```python
from build123d import *

# Parameters (mm, degrees)
BOSS_EXTRUDE1_DEPTH = 16
SKETCH4_R           = 11
BOSS_EXTRUDE5_DEPTH = 45
SKETCH8_R           = 12.5
BOSS_EXTRUDE8_DEPTH = 50
SKETCH11_R          = 12.5
CUT_EXTRUDE1_DEPTH  = 50
SKETCH12_R          = 17.5
CUT_EXTRUDE2_DEPTH  = 5
BOSS_EXTRUDE9_DEPTH = 6
RIB4_REACH          = 156.758
SKETCH16_WALL_W     = 366.24251427
SKETCH16_WALL_H     = 10


with BuildPart() as part:
    # Sketch2 → Boss-Extrude1 (new body)
    with BuildSketch(Plane(origin=(0, 0, 0), x_dir=(1, 0, 0), z_dir=(0, 1, 0))):
        with BuildLine():
            Line((0, 19), (0, 30))
            ThreePointArc((0, 30), (-30, 0), (0, -30))
            Line((0, -30), (0, -19))
            ThreePointArc((0, -19), (-19, 0), (0, 19))
        make_face()
    extrude(amount=BOSS_EXTRUDE1_DEPTH)



with BuildPart() as body_2:
    # Sketch4 → Boss-Extrude5 (new body)
    with BuildSketch(Plane(origin=(0, 0, 0), x_dir=(1, 0, 0), z_dir=(0, 1, 0))):
        with BuildLine():
            Line((-122.5, 25), (-105.941325388, 25))
            ThreePointArc((-105.941325388, 25), (-80.941325388, 0), (-105.941325388, -25))
            Line((-105.941325388, -25), (-122.5, -25))
            Line((-122.5, -25), (-122.5, 25))
        make_face()
        with Locations(Location((-105.941325388, 0, 0), (0, 0, 90))):
            Circle(SKETCH4_R, mode=Mode.SUBTRACT)
    extrude(amount=BOSS_EXTRUDE5_DEPTH)

    # Sketch8 → Boss-Extrude8 (add)
    with BuildSketch(Plane.XY.offset(25)):
        with Locations((-122.5, 22.5)):
            Circle(SKETCH8_R)
        with BuildLine():
            ThreePointArc((-122.5, 45), (-145, 22.5), (-122.5, 0))
            Line((-122.5, 0), (-122.5, 45))
        make_face()
        with BuildLine():
            ThreePointArc((-122.5, 35), (-135, 22.5), (-122.5, 10))
            Line((-122.5, 10), (-122.5, 35))
        make_face()
        with BuildLine():
            Line((-122.5, 35), (-122.5, 10))
            ThreePointArc((-122.5, 10), (-113.661165235, 13.661165235), (-110, 22.5))
            ThreePointArc((-110, 22.5), (-113.661165235, 31.338834765), (-122.5, 35))
        make_face()
    extrude(amount=-BOSS_EXTRUDE8_DEPTH)

    # Sketch11 → Cut-Extrude1 (cut)
    with BuildSketch(Plane.XY.offset(25)):
        with Locations((-122.5, 22.5)):
            Circle(SKETCH11_R)
    extrude(amount=-CUT_EXTRUDE1_DEPTH, mode=Mode.SUBTRACT)

    # Sketch12 → Cut-Extrude2 (cut)
    with BuildSketch(Plane.XY.offset(25)):
        with Locations((-122.5, 22.5)):
            Circle(SKETCH12_R)
    extrude(amount=-CUT_EXTRUDE2_DEPTH, mode=Mode.SUBTRACT)


with BuildPart() as part_1:
    add(part.part)

    add(body_2.part)  # Boss-Extrude9 merges body 2
    # Sketch13 → Boss-Extrude9 (add)
    with BuildSketch(Plane(origin=(0, 0, 0), x_dir=(1, 0, 0), z_dir=(0, 1, 0))):
        with BuildLine():
            ThreePointArc((-105.941325388, 25), (-80.941325388, 0), (-105.941325388, -25))
            Line((-105.941325388, -25), (-2.825462558, -29.86664965))
            ThreePointArc((-2.825462558, -29.86664965), (-30, 0), (-2.825462558, 29.86664965))
            Line((-2.825462558, 29.86664965), (-105.941325388, 25))
        make_face()
    extrude(amount=BOSS_EXTRUDE9_DEPTH)

    # Sketch16 wall → Rib4 (add, up to next)
    with BuildSketch(Plane(origin=(-55.470662694, 23, 0), x_dir=(0.930830223145, -0.365451906112, 0), z_dir=(0.365451906112, 0.930830223145, 0)), mode=Mode.PRIVATE) as rib4_sk1:
        Rectangle(SKETCH16_WALL_W, SKETCH16_WALL_H)
    rib4_tool1 = extrude(rib4_sk1.sketch, amount=-RIB4_REACH, mode=Mode.PRIVATE) - part_1.part
    add(rib4_tool1.solids().sort_by_distance((-55.470662694, 23, 0))[0])


solid = part_1.part
```
Build history of the part. All positions in model axes, mm. A direction names the side the tool comes from. Give positions to 0.01 mm unless a question says otherwise; leave off trailing zeros. Loops run counter-clockwise (first coordinate to the right, second up) from the corner with the lowest first, then second, coordinate; pieces in that order, holes last. Notation, with made-up numbers: (67.5, 35.25) -> (104.5, 35.25) arc R18 cw to (104.5, 50.25) -> close; hole circle Ø6 at (26, 31). An arc over 180 degrees is marked (long way). One line per question, with ' | ' between items.
Q1. Cut at D-D, the plane z = 12.5. Write the cut outline in (x, y), plus the area to 3 significant figures.
Filled sheet:
outline: (-122.5, 0) -> (-14.31, 0) -> (-14.31, 16) -> (-27.27, 16) -> (-27.27, 6) -> (-84.29, 6) -> (-84.29, 45) -> (-122.5, 45) arc R22.5 ccw to start; hole circle Ø25 at (-122.5, 22.5) | area: 2,570 mm²
Q2. Tool access for faces 4 (the flat face through (-134, 28, -25)), 5 (the flat face through (-55, 6, -18)), 6 (the cylindrical face through (-105.81, 27.76, 22.54)), 7 (the cylindrical face through (-82.267, 25.227, 8.032)), 8 (the flat face through (-58, 14, 5)): list every direction of +Z, -Z, +X, -X, +Y, -Y with a clear straight run to the whole face (end or side of a thin tool).
Filled sheet:
face 4: -Z, -X, +Y, -Y | face 5: -Z, +Y | face 6: +Z | face 7: +Y | face 8: +Z, +Y
Q3. Drop flat-ended pins along their axis: pin 1 (4 mm diameter, centred on y = 35.5, z = -2.5, fed in from -X); pin 2 (1 mm diameter, centred on y = 24.5, z = -23, fed in from +X); pin 3 (13.5 mm diameter, centred on x = -50.5, y = 13.5, fed in from +Z); pin 4 (15 mm diameter, centred on x = -122.5, y = 22.5, fed in from +Z). Give the stop position or say it passes through.
Filled sheet:
pin 1: stops at x = -142.13 | pin 2: stops at x = -95.04 | pin 3: stops at z = 5 | pin 4: passes through
Q4. Cut at A-A, the plane x = -125. Write the cut outline in (y, z).
Filled sheet:
outline: (0.14, -25) -> (10.25, -25) -> (10.25, 20) -> (5.18, 20) -> (5.18, 25) -> (0.14, 25) -> close; (34.75, -25) -> (44.86, -25) -> (44.86, 25) -> (39.82, 25) -> (39.82, 20) -> (34.75, 20) -> close
Q5. Cut at B-B, the plane y = 8.5. Write the cut outline in (x, z).
Filled sheet:
outline: (-140.11, -25) -> (-105.94, -25) arc R25 ccw to (-81.45, -5) -> (-29.58, -5) arc R30 ccw to (0, -30) -> (0, -19) arc R19 cw to (0, 19) -> (0, 30) arc R30 ccw to (-29.58, 5) -> (-81.45, 5) arc R25 ccw to (-105.94, 25) -> (-112, 25) -> (-112, 20) -> (-133, 20) -> (-133, 25) -> (-140.11, 25) -> close; hole circle Ø22 at (-105.94, 0)
Q6. Cut at C-C, the plane z = 0. Write the cut outline in (x, y).
Filled sheet:
outline: (-122.5, 0) -> (-116.94, 0) -> (-116.94, 11.3) arc R12.5 cw (long way) to (-116.94, 33.7) -> (-116.94, 45) -> (-122.5, 45) arc R22.5 ccw to start; (-94.94, 0) -> (-19, 0) -> (-19, 16) -> (-30, 16) -> (-30, 13) -> (-80.94, 33) -> (-80.94, 45) -> (-94.94, 45) -> close
Q7. Pull direction Y, two halves, no side cores. Call faces 1 (the cylindrical face through (-19, 8, 0)), 2 (the flat face through (-111, 15, 20)), 3 (the flat face through (-62, 0, 0)): pulls with the +Y half, pulls with the -Y half, needs draft (parallel to the pull), parting line crosses it, or undercut.
Filled sheet:
face 1: needs draft | face 2: undercut | face 3: pulls with the -Y half
Q8. Drill centre lines: line 1 along Y through (x, z) = (-123, -9.5); line 2 along Y through (x, z) = (-122.5, 21.6); line 3 along X through (y, z) = (12, 13.5). Where is each one in solid material? Low to high. Write a range as [from, to].
Filled sheet:
line 1: y = [0.01, 10.01], [34.99, 44.99] | line 2: y = [0, 5], [40, 45] | line 3: x = [-142.4, -129.28], [-115.72, -84.9], [-26.79, -13.37]
